Design review of the part built by this model. Coordinates are the model's own, in mm. Face numbers are marked on the shaded views. A direction names the side the tool comes from. Give positions to 0.01 mm unless a question says otherwise; leave off trailing zeros. Write each loop counter-clockwise with the first axis right and the second up, starting at its lowest first coordinate (ties: lowest second). Pieces come first, ordered by that corner, then holes. Notation, with made-up numbers: (-19.75, 71.25) -> (25.25, 71.25) arc R23 ccw to (25.25, 102.25) -> close; hole circle Ø5 at (66, -26.5). An arc over 180 degrees is marked (long way). Write each question's results on one line, items separated by ' | '. Start each with the question number.
(1) Take a section at B-B (x = 31.5). State the section outline as (y, z) points.
(2) Take a section at C-C (z = 35). State the section outline as (x, y) points, plus the area to 3 significant figures.
(3) Mouldability with a two-part tool opening along Z and no side actions: class the marked faces 1, 2 and 3 as released by +Z, released by -Z, zero draft, split by the parting line, or undercut.
(4) For the marked faces 4 and 5, list the 3-axis set-ups (+Z, -Z, +X, -X, +Y, -Y) from which the entire face can be reached by the end or side of a thin tool; tool diameter is ignored.
(5) To check wall thickness, follow probe 1 along Z at (x, y) = (10.25, 52.5); probe 2 along X at (y, z) = (5, 20); probe 3 along X at (y, z) = (28, 21). State the ranges of each line that lie inside material, in increasing order.
(6) Take a section at A-A (y = 14). State the section outline as (x, z) points, plus the area to 3 significant figures.
(7) Clearance check with flat-ended pins moving along their axes: pin 1 (2.5 mm diameter, centred on x = 11, z = 20, fed in from -Y); pin 2 (7.5 mm diameter, centred on y = 53.5, z = 14, fed in from -X); pin 3 (3.5 mm diameter, centred on y = 52.5, z = 10, fed in from +X). State where each tip first meets the part, or that it passes through.
(8) Take a section at D-D (y = 52.5). Count the separate pieces of the cut face and the enclosed holes in it, plus the area to 3 significant figures.
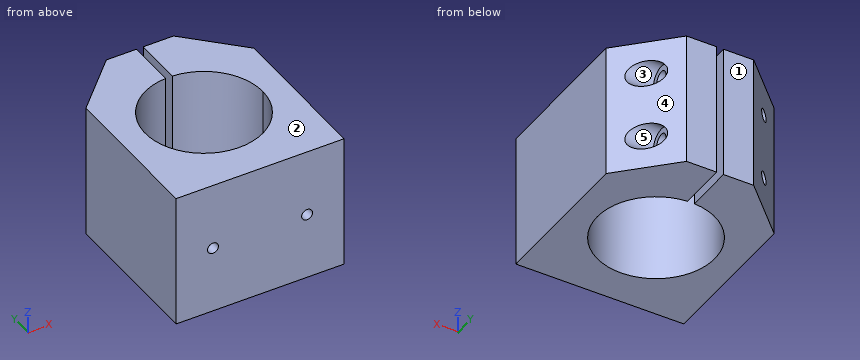
Autodesk Inventor part; units mm, degrees
ref_plane "Arbeitsebene1" through (42.5, 0, 0) normal (1, 0, 0) x (0, 0, -1)
ref_plane "Arbeitsebene3" through (0, 0, 30) normal (0, 0, 1) x (1, 0, 0)
ref_plane "Arbeitsebene4" through (0, 0, 10) normal (0, 0, -1) x (-1, 0, 0)
sketch "Skizze1" plane through (0, 0, 0) normal (0, 0, 1) x (1, 0, 0)
  line L0 (0, 0) -> (50, 0)
  line L1 (50, 0) -> (50, 45)
  line L2 (35, 60) -> (15, 60)
  line L3 (0, 45) -> (0, 0)
  circle A0 centre (25, 28) radius 17.5
  line L4 (25, 28) -> (25, 0) construction
  line L5 (0, 45) -> (15, 60)
  line L6 (35, 60) -> (50, 45)
  line L7 (24, 60) -> (26, 60)
  line L8 (26, 60) -> (26, 28)
  line L9 (26, 28) -> (24, 28)
  line L10 (24, 28) -> (24, 60)
  point P0 (50, 60)
  point P1 (0, 60)
  point P2 (25, 60)
  dimension "d0" = 50
  dimension "d1" = 35
  dimension "d2" = 60
  dimension "d3" = 15
  dimension "d4" = 15
  dimension "d5" = 15
  dimension "d6" = 15
  dimension "d7" = 28
  dimension "d10" = 2
extrude "Extrusion1" add sketch "Skizze1" along normal blind 40 contours L3 L5 L2 L10 A0 L8 L6 L1 L0 | L2 L8 A0 L10
extrude "Extrusion2" cut sketch "Skizze1" along normal up to surface (40 mm away) contours L2 L8 A0 L10 | A0 L8 L9 L10 picked at (24.8888, 33.8323)
sketch "Skizze2" plane through (0, 0, 0) normal (0, -1, 0) x (1, 0, 0)
  line L0 (0, 0) -> (0, 40) construction
  line L1 (50, 0) -> (50, 40) construction
  line L2 (0, 40) -> (50, 40) construction
  line L3 (0, 0) -> (0, 40) construction
  line L4 (25, 20) -> (25, 40) construction
  line L5 (7.5, 40) -> (42.5, 40) construction
  line L6 (11, 20) -> (39, 20) construction
  point P0 (26, 40)
  point P1 (24, 40)
  point P2 (0, 20)
  dimension "d13" = 28
hole "Bohrung1" at (11, 0, 20) at (39, 0, 20) direction (0, 1, 0) diameter 3.242 depth 11.8 tip angle 118
ref_plane "Arbeitsebene1" through (42.5, 0, 0) normal (1, 0, 0) x (0, 0, -1)
sketch "Skizze3" plane through (42.5, 0, 0) normal (1, 0, 0) x (0, 0, -1)
  line L0 (0, 60) -> (-40, 60) construction
  line L1 (0, 45) -> (-40, 45) construction
  line L2 (-40, 45) -> (-40, 60) construction
  line L3 (-40, 52.5) -> (0, 52.5) construction
  line L4 (0, 45) -> (0, 60) construction
  point P0 (0, 0)
  point P1 (-20, 52.5)
  point P2 (-30, 52.5)
  point P3 (-10, 52.5)
  dimension "d44" = 10
  dimension "d45" = 10
ref_plane "Arbeitsebene2" through (0, 0, 20) normal (0, 0, 1) x (1, 0, 0)
ref_plane "Arbeitsebene3" through (0, 0, 30) normal (0, 0, 1) x (1, 0, 0)
ref_plane "Arbeitsebene4" through (0, 0, 10) normal (0, 0, -1) x (-1, 0, 0)
sketch "Skizze5" plane through (50, 0, 40) normal (1, 0, 0) x (0, 0, -1)
  line L0 (20, -12) -> (20, 72) construction
  line L1 (10, -12) -> (10, 72) construction
  line L2 (30, 72) -> (30, -12) construction
  point P0 (40, 0)
  dimension "Hole_Dist2Center" = 10
  dimension "d37" = 10
hole "Bohrung2" at (42.5, 52.5, 30) at (42.5, 52.5, 10) direction (-1, 0, 0) diameter 4.5 depth 18.5 counterbore diameter 8 counterbore depth 4.5
delete faces "Fläche löschen1" heal yes whole lump no faces at (42.5, 52.1809, 31.2946) (42.5, 50.9777, 9.002)
sketch "Skizze4" plane through (24, 45.4714, 0) normal (1, 0, 0) x (0, 0, -1)
  line L0 (-20, 7.0286) -> (-30, 7.0286) construction
  line L1 (-30, -57.4714) -> (-30, 26.5286) construction
  line L2 (-10, 26.5286) -> (-10, -57.4714) construction
  point P0 (0, -45.4714)
  point P1 (-10, 7.0286)
hole "Bohrung3" at (24, 52.5, 30) at (24, 52.5, 10) direction (-1, 0, 0) diameter 3.242 end through all
equation "\"d0\" = Fixation_Width"
equation "\"d8\" = Fixation_Thickness"
equation "\"d11\" = Fixation_Thickness"
equation "\"d13\" = FixationHole_Dist"
equation "\"Fixation_Thickness\" = 40"
equation "\"Fixation_Width\" = 50"
equation "\"FixationHole_Dist\" = 28"
equation "\"d21\" = -0.5 * d5"
properties part number "Motor_MainAxis_Fixation_Holder"
Report:
1) outline: (0, 0) -> (11.75, 0) -> (11.75, 40) -> (0, 40) -> close; (44.25, 0) -> (60, 0) -> (60, 40) -> (44.25, 40) -> close; hole circle Ø4.5 at (52.5, 10); hole circle Ø4.5 at (52.5, 30)
2) outline: (0, 0) -> (50, 0) -> (50, 45) -> (35, 60) -> (26, 60) -> (26, 45.47) arc R17.5 cw (long way) to (24, 45.47) -> (24, 60) -> (15, 60) -> (0, 45) -> close | area: 1,780 mm2
3) face 1: zero draft | face 2: released by +Z | face 3: undercut
4) face 4: +Z, -Z, +X, +Y | face 5: +X
5) probe 1: 0 to 8.38, 11.62 to 28.38, 31.62 to 40 | probe 2: 0 to 9.38, 12.62 to 37.38, 40.62 to 50 | probe 3: 0 to 7.5, 42.5 to 50
6) outline: (0, 0) -> (14.5, 0) -> (14.5, 40) -> (0, 40) -> close; (35.5, 0) -> (50, 0) -> (50, 40) -> (35.5, 40) -> close | area: 1,160 mm2
7) pin 1: y = 12.02 | pin 2: x = 4.75 | pin 3: x = 24
8) separate pieces: 6 | enclosed holes: 0 | area: 1,030 mm2
